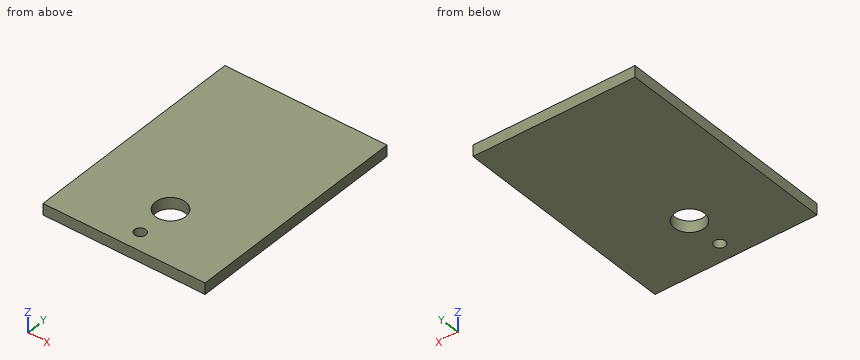
```python
from build123d import *

# Parameters (mm, degrees)
SKETCH1_W           = 1092.2
SKETCH1_H           = 1524
SKETCH1_R           = 101.6
SKETCH1_R_2         = 38.1
BOSS_EXTRUDE1_DEPTH = 76.2


with BuildPart() as part:
    # Sketch1 → Boss-Extrude1 (new body)
    with BuildSketch(Plane.XY):
        with Locations((546.1, 762)):
            Rectangle(SKETCH1_W, SKETCH1_H)
        with Locations(Location((552.718036359, 381, 0), (0, 0, 180))):
            Circle(SKETCH1_R, mode=Mode.SUBTRACT)
        with Locations(Location((552.718036359, 127, 0), (0, 0, 180))):
            Circle(SKETCH1_R_2, mode=Mode.SUBTRACT)
    extrude(amount=BOSS_EXTRUDE1_DEPTH)


solid = part.part
```
Read the model definition and answer for the solid it produces. Units are mm, in the model's axes. Coordinates: 2 decimals unless noted, no trailing zeros. Loops run counter-clockwise (first coordinate to the right, second up) from the corner with the lowest first, then second, coordinate; pieces in that order, holes last. Notation, with made-up numbers: (-26, -4) -> (-6, -4) arc R12 cw to (-6, 17) -> close; hole circle Ø6 at (28.5, 3). An arc over 180 degrees is marked (long way). Return JSON: item names as keys, results as strings.
Item 1: A flat-ended cylindrical pin translates along its axis: P1, Ø2, axis at y = 1086, z = 32.5, coming from the -X side. Find the tip coordinate at first contact, or state that the pin passes through.
Answers:
{"P1": "stops at x = 0"}
Item 2: Find the intervals of material crossed by probe 1 along Y at (x, z) = (581.5, 46); probe 2 along Y at (x, z) = (541.5, 14.5); probe 3 along X at (y, z) = (378.5, 23), in increasing order.
Answers:
{"probe 1": "y = 0 to 102.04, 151.96 to 283.56, 478.44 to 1524", "probe 2": "y = 0 to 90.59, 163.41 to 280.02, 481.98 to 1524", "probe 3": "x = 0 to 451.15, 654.29 to 1092.2"}
Item 3: Find section D-D (y = 381). Determine the outline of the cut face in (x, z), plus the area to 3 significant figures.
Answers:
{"outline": "(0, 0) -> (451.12, 0) -> (451.12, 76.2) -> (0, 76.2) -> close; (654.32, 0) -> (1092.2, 0) -> (1092.2, 76.2) -> (654.32, 76.2) -> close", "area": "67,700 mm2"}
Item 4: Find section B-B (z = 36.5). Determine the outline of the cut face in (x, y).
Answers:
{"outline": "(0, 0) -> (1092.2, 0) -> (1092.2, 1524) -> (0, 1524) -> close; hole circle Ø203.2 at (552.72, 381); hole circle Ø76.2 at (552.72, 127)"}
Item 5: Find section A-A (y = 127). Determine the outline of the cut face in (x, z), plus the area to 3 significant figures.
Answers:
{"outline": "(0, 0) -> (514.62, 0) -> (514.62, 76.2) -> (0, 76.2) -> close; (590.82, 0) -> (1092.2, 0) -> (1092.2, 76.2) -> (590.82, 76.2) -> close", "area": "77,400 mm2"}
Item 6: Find section C-C (x = 567.5). Determine the outline of the cut face in (y, z), plus the area to 3 significant figures.
Answers:
{"outline": "(0, 0) -> (91.88, 0) -> (91.88, 76.2) -> (0, 76.2) -> close; (162.12, 0) -> (280.48, 0) -> (280.48, 76.2) -> (162.12, 76.2) -> close; (481.52, 0) -> (1524, 0) -> (1524, 76.2) -> (481.52, 76.2) -> close", "area": "95,500 mm2"}
